from build123d import *

# Parameters (mm, degrees)
F0_R      = 8.5
F1_DEPTH  = 140
F2_R      = 6
F3_DEPTH  = 30
F4_W      = 9
F4_H      = 9
F5_DEPTH  = 11
F6_SIZE   = 0.5
F7_SIZE   = 0.5
F8_SIZE   = 0.5
F9_R      = 1.65
F10_DEPTH = 25
F11_R     = 8.5
F11_R_2   = 6
F12_DEPTH = 40
F14_DEPTH = 11


# Not quite as in the source:
# - a pattern or mirror of a feature is missing from the dataset's text; its kind, count and spacing are read off the source's solid


with BuildPart() as f1:
    # F0 (on Front) → F1 (new body)
    with BuildSketch(Plane.XZ):
        Circle(F0_R)
    extrude(amount=F1_DEPTH)

    # F2 (on face) → F3 (cut)
    with BuildSketch(Plane.XZ.offset(140)):
        Circle(F2_R)
    extrude(amount=-F3_DEPTH, mode=Mode.SUBTRACT)

    # F4 (on face) → F5 (cut)
    with BuildSketch(Plane.XZ.offset(110)):
        Rectangle(F4_W, F4_H)
    extrude(amount=-F5_DEPTH, mode=Mode.SUBTRACT)

    # F6
    f6_edges = [f1.edges().sort_by_distance(p)[0] for p in [
        (-4.5, -104.5, -4.5),
    ]]
    chamfer(f6_edges, length=F6_SIZE)

    # F7
    f7_edges = [f1.edges().sort_by_distance(p)[0] for p in [
        (4.5, -104.5, -4.5),
    ]]
    chamfer(f7_edges, length=F7_SIZE)

    # F8
    f8_edges = [f1.edges().sort_by_distance(p)[0] for p in [
        (4.5, -104.5, 4.5),
        (-4.5, -104.5, 4.5),
    ]]
    chamfer(f8_edges, length=F8_SIZE)

    # F9 (on face) → F10 (cut)
    with BuildSketch(Plane.YZ.offset(-4.5)):
        with Locations((-104, 0)):
            Circle(F9_R)
    f10 = extrude(amount=-F10_DEPTH, mode=Mode.SUBTRACT)

    # F10_copies: F10 across plane
    add(f10.mirror(Plane(origin=(5.8e-05, 0, 0), x_dir=(1e-06, 1, 0), z_dir=(1, -1e-06, 0))), mode=Mode.SUBTRACT)

    # F11 (on face) → F12 (cut)
    with BuildSketch(Plane(origin=(0, 0, 0), x_dir=(-1, 0, 0), z_dir=(0, 1, 0))):
        Circle(F11_R)
        Circle(F11_R_2, mode=Mode.SUBTRACT)
    extrude(amount=-F12_DEPTH, mode=Mode.SUBTRACT)

    # F13 (on face) → F14 (cut)
    with BuildSketch(Plane(origin=(0, 0, 0), x_dir=(-1, 0, 0), z_dir=(0, 1, 0))):
        with BuildLine():
            Line((3.9686269666, -4.5), (-3.9686269666, -4.5))
            ThreePointArc((-3.9686269666, -4.5), (0, -6), (3.9686269666, -4.5))
        make_face()
        with BuildLine():
            ThreePointArc((-4.5, 3.9686269666), (-6, 0), (-4.5, -3.9686269666))
            Line((-4.5, -3.9686269666), (-4.5, 3.9686269666))
        make_face()
        with BuildLine():
            Line((-4.5, 4.5), (-4.5, 3.9686269666))
            ThreePointArc((-4.5, 3.9686269666), (-4.2426406871, 4.2426406871), (-3.9686269666, 4.5))
            Line((-3.9686269666, 4.5), (-4.5, 4.5))
        make_face()
        with BuildLine():
            Line((4.5, 3.9686269666), (4.5, -3.9686269666))
            ThreePointArc((4.5, -3.9686269666), (5.6124860802, -2.1213203436), (6, 0))
            ThreePointArc((6, 0), (5.6124860802, 2.1213203436), (4.5, 3.9686269666))
        make_face()
        with BuildLine():
            ThreePointArc((3.9686269666, 4.5), (0, 6), (-3.9686269666, 4.5))
            Line((-3.9686269666, 4.5), (3.9686269666, 4.5))
        make_face()
        with BuildLine():
            ThreePointArc((3.9686269666, 4.5), (4.2426406871, 4.2426406871), (4.5, 3.9686269666))
            Line((4.5, 3.9686269666), (4.5, 4.5))
            Line((4.5, 4.5), (3.9686269666, 4.5))
        make_face()
    extrude(amount=-F14_DEPTH, mode=Mode.SUBTRACT)


solid = f1.part
Design review of the part built by this model. Coordinates are the model's own, in mm. A direction names the side the tool comes from. Round coordinates to 2 decimals unless told otherwise and drop trailing zeros. Write each loop counter-clockwise with the first axis right and the second up, starting at its lowest first coordinate (ties: lowest second). Pieces come first, ordered by that corner, then holes.
Item 1: Consider section C-C on y = -130. Give the boundary of the cut face in (x, z), and give its area (3 significant figures).
Item 2: For pin 1 Ø0.7 at (x, z) = (1.5, -5) entering from +Y; pin 2 Ø8.5 at (y, z) = (-6.5, 1) entering from -X; pin 3 Ø5 at (x, y) = (4, -107.5) entering from +Z, all flat-tipped, find the tip position at first contact; note any pin that passes through.
Item 3: Wall thickness on L1, parallel to Z at x = 0, y = -133.5; L2, parallel to Z at x = 0.5, y = -105.5; L3, parallel to Y at x = 5.7, z = 0: over which ranges is each line inside the solid? List them lowest first.
Item 4: Consider section D-D on y = -54. Give the boundary of the cut face in (x, z).
Item 5: Consider section A-A on z = 0. Give the boundary of the cut face in (x, y), and give its area (3 significant figures).
Item 6: Draft analysis for pull direction X (two halves, no side actions). For faces 1 (the flat face through (0, -5, -4.5)), 2 (the flat face through (0, -105, 4.5)), 3 (the flat face through (4.5, -5, 0)), state which applies: released by +X, released by -X, zero draft, split by the parting line, or undercut.
Item 7: Consider section B-B on x = 0. Give the boundary of the cut face in (y, z).
Item 8: For faces 4 (the flat face through (4.5, -106, 0)), 5 (the flat face through (-4.5, -5, 0)), 6 (the flat face through (0, -5, 4.5)), 7 (the flat face through (-2, -40, 6)), list the 3-axis set-ups (+Z, -Z, +X, -X, +Y, -Y) from which the entire face can be reached by the end or side of a thin tool; tool diameter is ignored.
Check values:
1. outline: circle Ø17 at (0, 0); hole circle Ø12 at (0, 0)
1. area: 114 mm2
2. pin 1: stops at y = -11
2. pin 2: stops at x = -4.5
2. pin 3: stops at z = 8.37
3. L1: z = -8.5 to -6, 6 to 8.5
3. L2: z = -8.49 to -4.5, 4.5 to 8.49
3. L3: y = -110 to -105.65, -102.35 to -11
4. outline: circle Ø17 at (0, 0)
5. outline: (-8.5, -140) - (-6, -140) - (-6, -110) - (-4.5, -110) - (-4.5, -105.65) - (-8.5, -105.65) - close; (-8.5, -102.35) - (-4.5, -102.35) - (-4.5, -99) - (4.5, -99) - (4.5, -102.35) - (8.5, -102.35) - (8.5, -40) - (6, -40) - (6, -11) - (4.5, -11) - (4.5, 0) - (-4.5, 0) - (-4.5, -11) - (-6, -11) - (-6, -40) - (-8.5, -40) - close; (4.5, -110) - (6, -110) - (6, -140) - (8.5, -140) - (8.5, -105.65) - (4.5, -105.65) - close
5. area: 1,660 mm2
6. face 1: zero draft
6. face 2: undercut
6. face 3: released by +X
7. outline: (-140, -8.5) - (-40, -8.5) - (-40, -6) - (-11, -6) - (-11, -4.5) - (0, -4.5) - (0, 4.5) - (-11, 4.5) - (-11, 6) - (-40, 6) - (-40, 8.5) - (-140, 8.5) - (-140, 6) - (-110, 6) - (-110, 4.5) - (-99, 4.5) - (-99, -4.5) - (-110, -4.5) - (-110, -6) - (-140, -6) - close
8. face 4: -Y
8. face 5: +Z, -Z, -X, +Y
8. face 6: +Z, +X, -X, +Y
8. face 7: +Y
